```python
from build123d import *


with BuildPart() as part:
    # Sketch1 → Revolve1 (revolve)
    with BuildSketch(Plane(origin=(0, 0, 0), x_dir=(0, 0, -1), z_dir=(1, 0, 0))):
        Polygon((-1.4986, 2.413), (-1.4986, 3.3401), (0, 3.3401), (0, 5.08), (0.254, 5.08), (0.254, 5.5324375), (1.27, 6.5484375), (10.3632, 6.5484375), (11.3792, 5.5324375), (11.3792, 0), (-11.1252, 0), (-11.1252, 1.357141828), (-10.5156, 2.413), align=None)
    revolve(axis=Axis((0, 0, 11.1252), (0, 0, 1)))


solid = part.part
```
Work out the finished part from the listing and answer in its coordinate system (mm). A direction names the side the tool comes from. Coordinates: 2 decimals unless noted, no trailing zeros. Order: outer loops, then holes, each group sorted by start corner. A loop starts at its lowest first (then second) coordinate and runs counter-clockwise, first axis right, second up. Notation, with made-up numbers: M 23,-14 L 43,-14 A26 cw 43,8 Z; hole C 20,30 d2. An arc over 180 degrees is marked long. Use CSV: the item, a comma, the result in double quotes.
1) For faces 1 (the face through (3.3, 1.2, 0)), 2 (the face through (6.393, -1.42, -5.88)), determine the directions among +Z, -Z, +X, -X, +Y, -Y from which every point of the face is accessible in a straight line to the end or side of a thin tool.
Worked out:
face 1,"+Z"
face 2,"+Z, -Z"
2) Section C-C on z = 0.5 is taken. Write down the section's boundary in (x, y), plus the area to 3 significant figures.
Worked out:
outline,"C 0,0 d6.68"
area,"35.0 mm^2"
3) Flat-ended cylindrical pins translate along their axes: pin 1 Ø1 at (y, z) = (3, -2.5) entering from +X; pin 2 Ø1 at (x, y) = (3.5, -5) entering from -Z; pin 3 Ø3.5 at (x, y) = (2.5, 2.5) entering from +Z. Find the tip coordinate at first contact, or state that the pin passes through.
Worked out:
pin 1,"stops at x = 6.05"
pin 2,"stops at z = -11.31"
pin 3,"stops at z = 10.88"
4) Section A-A on y = 0 is taken. Write down the section's boundary in (x, z).
Worked out:
outline,"M -6.55,-10.36 L -5.53,-11.38 L 5.53,-11.38 L 6.55,-10.36 L 6.55,-1.27 L 5.53,-0.25 L 5.08,-0.25 L 5.08,0 L 3.34,0 L 3.34,1.5 L 2.41,1.5 L 2.41,10.52 L 1.36,11.13 L -1.36,11.13 L -2.41,10.52 L -2.41,1.5 L -3.34,1.5 L -3.34,0 L -5.08,0 L -5.08,-0.25 L -5.53,-0.25 L -6.55,-1.27 Z"
5) Consider line 1 (Z direction, x = 0, y = -3.25); line 2 (Z direction, x = 4.25, y = 1.75); line 3 (Y direction, x = -4.25, z = -1.5). Determine where each line is inside the solid, lowest interval first. Write a range as [from, to].
Worked out:
line 1,"z = [-11.38, 1.5]"
line 2,"z = [-11.38, 0]"
line 3,"y = [-4.98, 4.98]"
6) Section D-D on z = -9.5 is taken. Write down the section's boundary in (x, y).
Worked out:
outline,"C 0,0 d13.1"
